```python
from build123d import *

# Parameters (mm, degrees)
EXTRUDE_1_DEPTH     = 20
SKETCH_3_OUTSIDE_W  = 62.49
SKETCH_3_OUTSIDE_H  = 56.148
SKETCH_3_OUTSIDE_R  = 18.45
CUT_EXTRUDE_1_DEPTH = 12
SKETCH_11_R         = 16.7
CUT_EXTRUDE_2_DEPTH = 1.5
SKETCH_13_R         = 15
CUT_EXTRUDE_4_DEPTH = 17
SKETCH_14_R         = 15.7
CUT_EXTRUDE_5_DEPTH = 13.5
SKETCH_15_W         = 1
SKETCH_15_H         = 9
SKETCH_16_R         = 6.2
EXTRUDE_2_DEPTH     = 2.5
SKETCH_17_R         = 6.95
EXTRUDE_3_DEPTH     = 7.9
SKETCH_18_R         = 6.2
EXTRUDE_4_DEPTH     = 2
SKETCH_21_R         = 2.85
CUT_EXTRUDE_6_DEPTH = 49.016073698


with BuildPart() as part:
    # Эскиз2 → Бобышка-Вытянуть1 (new body)
    with BuildSketch(Plane(origin=(0, 0, 0), x_dir=(1, 0, 0), z_dir=(0, 1, 0))):
        Polygon((11.835680518, -20.5), (23.671361037, 0), (11.835680518, 20.5), (-11.835680518, 20.5), (-23.671361037, 0), (-11.835680518, -20.5), align=None)
    extrude(amount=EXTRUDE_1_DEPTH)

    # Эскиз3 outside → Вырез-Вытянуть1 (cut)
    with BuildSketch(Plane.XZ):
        Rectangle(SKETCH_3_OUTSIDE_W, SKETCH_3_OUTSIDE_H)
        with Locations(Location((0, 0, 0), (0, 0, 270))):
            Circle(SKETCH_3_OUTSIDE_R, mode=Mode.SUBTRACT)
    extrude(amount=-CUT_EXTRUDE_1_DEPTH, mode=Mode.SUBTRACT)

    # Эскиз10 → Вырез-Повернуть1 (revolve, cut)
    with BuildSketch(Plane.XY):
        Polygon((23.671361037, 20), (23.671361037, 19), (20.5, 20), align=None)
    cut_revolve_1 = revolve(axis=Axis((0, 12, 0), (0, -1, 0)), mode=Mode.SUBTRACT)

    # Зеркальное отражение1: Вырез-Повернуть1 across plane
    add(cut_revolve_1.mirror(Plane(origin=(0, 16, 0), x_dir=(0, 0, 1), z_dir=(0, -1, 0))), mode=Mode.SUBTRACT)

    # Эскиз11 → Вырез-Вытянуть2 (cut)
    with BuildSketch(Plane.XZ):
        with Locations(Location((0, 0, 0), (0, 0, 270))):
            Circle(SKETCH_11_R)
    extrude(amount=-CUT_EXTRUDE_2_DEPTH, mode=Mode.SUBTRACT)

    # Эскиз13 → Вырез-Вытянуть4 (cut)
    with BuildSketch(Plane.XZ):
        with Locations(Location((0, 0, 0), (0, 0, 270))):
            Circle(SKETCH_13_R)
    extrude(amount=-CUT_EXTRUDE_4_DEPTH, mode=Mode.SUBTRACT)

    # Эскиз14 → Вырез-Вытянуть5 (cut)
    with BuildSketch(Plane(origin=(0, 3.5, 0), x_dir=(-1, 0, 0), z_dir=(0, -1, 0))):
        with Locations(Location((0, 0, 0), (0, 0, 90))):
            Circle(SKETCH_14_R)
    extrude(amount=-CUT_EXTRUDE_5_DEPTH, mode=Mode.SUBTRACT)

    # Эскиз15 → Повернуть1 (revolve)
    with BuildSketch(Plane.XY, mode=Mode.PRIVATE) as revolve_1_sk:
        with Locations((18.95, 4.5)):
            Rectangle(SKETCH_15_W, SKETCH_15_H)
    revolve(revolve_1_sk.sketch.rotate(Axis((0, 17, 0), (0, -1, 0)), 90), axis=Axis((0, 17, 0), (0, -1, 0)))

    # Эскиз16 → Бобышка-Вытянуть2 (add)
    with BuildSketch(Plane(origin=(0, 20, 0), x_dir=(1, 0, 0), z_dir=(0, 1, 0))):
        with Locations(Location((0, 0, 0), (0, 0, 270))):
            Circle(SKETCH_16_R)
    extrude(amount=EXTRUDE_2_DEPTH)

    # Эскиз17 → Бобышка-Вытянуть3 (add)
    with BuildSketch(Plane(origin=(0, 22.5, 0), x_dir=(1, 0, 0), z_dir=(0, 1, 0))):
        with Locations(Location((0, 0, 0), (0, 0, 270))):
            Circle(SKETCH_17_R)
    extrude(amount=EXTRUDE_3_DEPTH)

    # Эскиз18 → Бобышка-Вытянуть4 (add)
    with BuildSketch(Plane(origin=(0, 30.4, 0), x_dir=(1, 0, 0), z_dir=(0, 1, 0))):
        with Locations(Location((0, 0, 0), (0, 0, 270))):
            Circle(SKETCH_18_R)
    extrude(amount=EXTRUDE_4_DEPTH)

    # Эскиз19 → Повернуть2 (revolve)
    with BuildSketch(Plane.XY):
        Polygon((6.2, 32.4), (2.85, 36.4), (0, 36.4), (0, 32.4), align=None)
    revolve(axis=Axis((0, -964.782676563, 0), (0, 1, 0)))

    # Эскиз21 → Вырез-Вытянуть6 (cut, through all)
    with BuildSketch(Plane(origin=(0, 36.4, 0), x_dir=(1, 0, 0), z_dir=(0, 1, 0))):
        with Locations(Location((0, 0, 0), (0, 0, 180))):
            Circle(SKETCH_21_R)
    extrude(amount=-CUT_EXTRUDE_6_DEPTH, mode=Mode.SUBTRACT)

    # Эскиз22 → Вырез-Повернуть2 (revolve, cut)
    with BuildSketch(Plane.XY, mode=Mode.PRIVATE) as cut_revolve_2_sk:
        Polygon((0, 20.123304437), (5.409721973, 17), (0, 17), align=None)
    revolve(cut_revolve_2_sk.sketch.rotate(Axis((0, 17, 0), (0, 1, 0)), 180), axis=Axis((0, 17, 0), (0, 1, 0)), mode=Mode.SUBTRACT)


solid = part.part
```
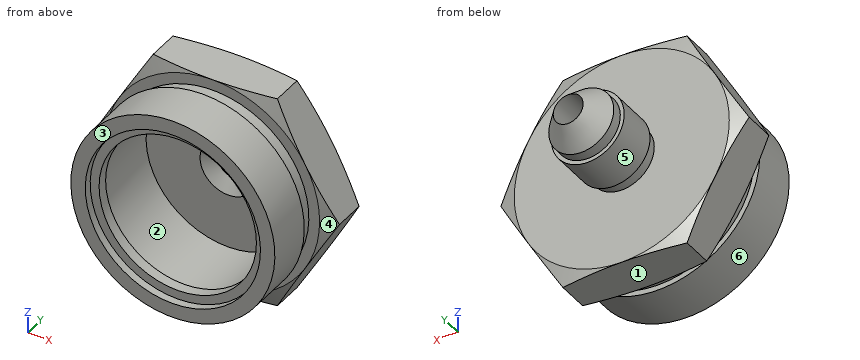
Build history of the part. All positions in model axes, mm. Face numbers are marked on the shaded views. A direction names the side the tool comes from. Give positions to 0.01 mm unless a question says otherwise; leave off trailing zeros. Loops run counter-clockwise (first coordinate to the right, second up) from the corner with the lowest first, then second, coordinate; pieces in that order, holes last. Notation, with made-up numbers: (4.5, -22.5) - (41.5, -22.5) arc R35 ccw to (41.5, 15.5) - close; hole circle Ø7 at (85, -20). An arc over 180 degrees is marked (long way). Use a Markdown table: item, result.
(1) Wall check: line 1 along Y through (x, z) = (15, -11); line 2 along X through (y, z) = (27, 0); line 3 along Y through (x, z) = (15, 3.5). Give the ranges that are in metal, low to high.
Taken from the geometry:
| item | result |
|---|---|
| line 1 | 0 to 9, 12 to 20 |
| line 2 | -6.95 to -2.85, 2.85 to 6.95 |
| line 3 | 1.5 to 3.5, 17 to 20 |
(2) Which spindle directions (+Z, -Z, +X, -X, +Y, -Y) get a long thin tool onto all of the face, cutting with end or side? Do the marked faces 4, 5 and 6. Say none if no direction does.
Taken from the geometry:
| item | result |
|---|---|
| face 4 | +X, -Y |
| face 5 | +Y |
| face 6 | -Y |
(3) Drop flat-ended pins along their axis: pin 1 Ø11 at (x, z) = (3.5, -2.5) entering from -Y; pin 2 Ø11 at (x, z) = (1.5, -1) entering from +Y; pin 3 Ø12 at (y, z) = (17, 10.5) entering from -X; pin 4 Ø4 at (x, z) = (0, -7) entering from +Y. Give the stop position or say it passes through.
Taken from the geometry:
| item | result |
|---|---|
| pin 1 | y = 17 |
| pin 2 | y = 36.4 |
| pin 3 | x = -21.07 |
| pin 4 | y = 33.83 |
(4) Pull direction Z, two halves, no side cores. Call the marked faces 1, 2 and 3: +Z half, -Z half, draft (parallel to the pull), parting line (faces both ways), or undercut.
Taken from the geometry:
| item | result |
|---|---|
| face 1 | -Z half |
| face 2 | undercut |
| face 3 | draft |
(5) Band-saw the part on A-A (y = 16). Give the cut face in (x, z).
Taken from the geometry:
| item | result |
|---|---|
| outline | (-23.67, 0) - (-11.84, -20.5) - (11.84, -20.5) - (23.67, 0) - (11.84, 20.5) - (-11.84, 20.5) - close; hole circle Ø31.4 at (0, 0) |
(6) Band-saw the part on C-C (y = 5.5). Give the cut face in (x, z), and give its area (3 significant figures).
Taken from the geometry:
| item | result |
|---|---|
| outline | circle Ø38.9 at (0, 0); hole circle Ø31.4 at (0, 0) |
| area | 414 mm2 |
(7) Band-saw the part on B-B (y = 21). Give the cut face in (x, z).
Taken from the geometry:
| item | result |
|---|---|
| outline | circle Ø12.4 at (0, 0); hole circle Ø5.7 at (0, 0) |
